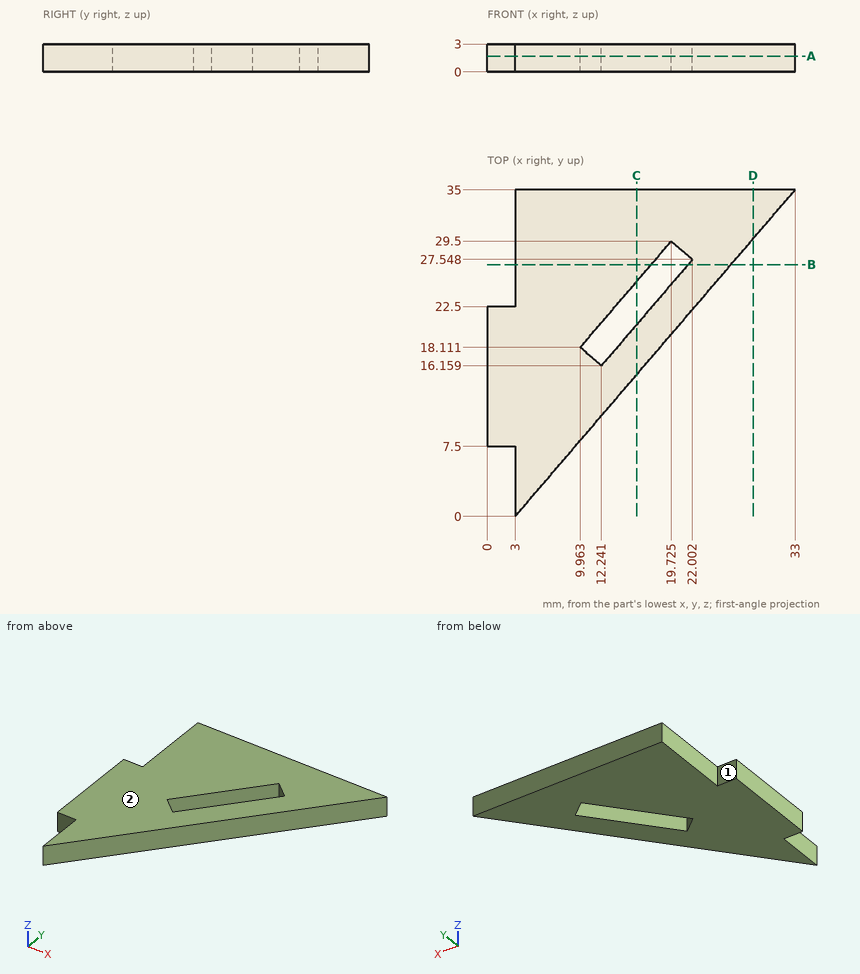
Verification items for this drawing (mm, ordinates from the low corner). A direction names the side the tool comes from. Coordinates: 2 decimals unless noted, no trailing zeros. Order: outer loops, then holes, each group sorted by start corner. A loop starts at its lowest first (then second) coordinate and runs counter-clockwise, first axis right, second up. Notation, with made-up numbers: (67, 55) - (103, 55) arc R9 ccw to (103, 66) - close; hole circle Ø4 at (-3.75, 74.5). An arc over 180 degrees is marked (long way). Answer in a Markdown table with one row per item. Add a question column.
1. Section check C-C (x = 16). Enter the section's corners in (y, z) (1 decimal).
2. Material ranges on L1, parallel to X at y = 27.5, z = 2.85; L2, parallel to X at y = 28, z = 1.6 (1 decimal); L3, parallel to Y at x = 15, z = 2.55 (1 decimal), recorded low to high. Write a range as [from, to].
3. Access from +Z, -Z, +X, -X, +Y, -Y to the whole of each face (thin tool, end or side, straight path). Record for the marked faces 1 and 2.
4. Section check D-D (x = 28.5). Enter the section's corners in (y, z).
5. Section check A-A (z = 1.7). Enter the section's corners in (x, y) (1 decimal).
6. Section check B-B (y = 27). Enter the section's corners in (x, z).
7. Gauge pin test, flat ends, axial feed: pin 1 Ø12 at (x, y) = (23, 22.5) entering from -Z; pin 2 Ø1.5 at (x, z) = (1, 2) entering from -Y. Record the tip position at first contact, or that the pin passes through.
Data:
| question | item | result |
|---|---|---|
| 1 | outline | (15.2, 0) - (20.5, 0) - (20.5, 3) - (15.2, 3) - close; (25.2, 0) - (35, 0) - (35, 3) - (25.2, 3) - close |
| 2 | L1 | x = [3, 18.01], [21.96, 26.57] |
| 2 | L2 | x = [3, 18.4], [21.5, 27] |
| 2 | L3 | y = [14, 19.4], [24, 35] |
| 3 | face 1 | +Z, -Z, -X, +Y |
| 3 | face 2 | +Z, +X, -X, +Y, -Y |
| 4 | outline | (29.75, 0) - (35, 0) - (35, 3) - (29.75, 3) - close |
| 5 | outline | (0, 7.5) - (3, 7.5) - (3, 0) - (33, 35) - (3, 35) - (3, 22.5) - (0, 22.5) - close; hole (10, 18.1) - (12.2, 16.2) - (22, 27.5) - (19.7, 29.5) - close |
| 6 | outline | (3, 0) - (17.58, 0) - (17.58, 3) - (3, 3) - close; (21.53, 0) - (26.14, 0) - (26.14, 3) - (21.53, 3) - close |
| 7 | pin 1 | stops at z = 0 |
| 7 | pin 2 | stops at y = 7.5 |
